Here's how the part is built. I have some questions about the finished solid (model axes, mm). Face numbers are marked on the shaded views. A direction names the side the tool comes from. Coordinates: 2 decimals unless noted, no trailing zeros. Loops run counter-clockwise (first coordinate to the right, second up) from the corner with the lowest first, then second, coordinate; pieces in that order, holes last. Notation, with made-up numbers: (-36.75, -16) -> (7.25, -16) arc R23 cw to (7.25, -4) -> close; hole circle Ø6 at (21.5, 50.5). An arc over 180 degrees is marked (long way). Use CSV: the item, a comma, the result in double quotes. Start each with the question number.
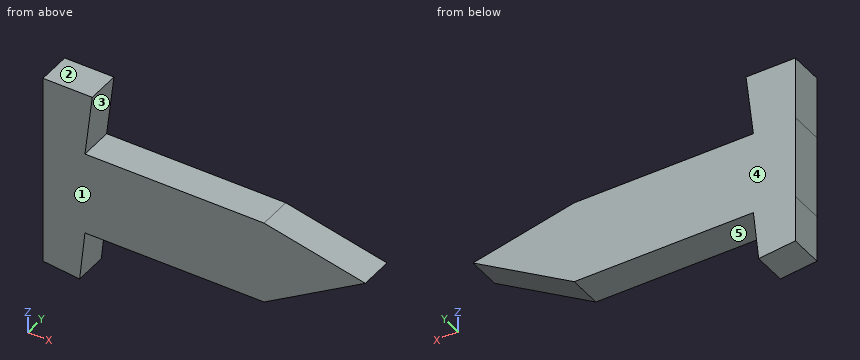
from build123d import *

# Parameters (mm, degrees)
F0_W     = 31.524651
F0_H     = 62.468918
F0_W_2   = 134.60525
F1_DEPTH = 25.4


with BuildPart() as f1:
    # F0 (on Front) → F1 (new body)
    with BuildSketch(Plane.XZ):
        with Locations((-136.606816, -14.502092)):
            Rectangle(F0_W, F0_H)
        Polygon((-120.844491, -45.736551), (-152.369142, -45.736551), (-152.369142, -80.935445), (-124.847621, -83.827771), align=None)
        with Locations((-53.541866, -14.502092)):
            Rectangle(F0_W_2, F0_H)
        Polygon((-152.369142, 63.859507), (-152.369142, 16.732367), (-120.844491, 16.732367), (-115.340188, 63.859507), align=None)
        Polygon((13.760759, 16.732367), (13.760759, -45.736551), (89.820236, 0), align=None)
    extrude(amount=F1_DEPTH)


solid = f1.part
1) I want a section at A-A, the plane y = -4.75. Please give me the cut outline in (x, z), plus the area to 3 significant figures.
2) Thinking about a two-plate mould opening in Z: for the marked faces 1, 2 and 3, which applies, pulls with the +Z half, pulls with the -Z half, needs draft (parallel to the pull), parting line crosses it, or undercut?
3) Which directions (+Z, -Z, +X, -X, +Y, -Y) give clear straight access to the entire face, cutting with the end or side of a thin tool? Please do the marked faces 4 and 5.
4) I want a section at B-B, the plane x = -40.5. Please give me the cut outline in (y, z), plus the area to 3 significant figures.
5) I want a section at C-C, the plane z = 12. Please give me the cut outline in (x, y), plus the area to 3 significant figures.
6) For P1, Ø4, axis at x = -51.5, y = -18, coming from the -Z side; P2, Ø1, axis at y = -14, z = -21, coming from the +X side; P3, Ø12, axis at y = -20, z = -9.5, coming from the +X side, each with a flat end and sliding along its axis, tell me the tip position at first contact or that it passes through.
7) Please list where these lines run through material, in increasing order: L1, parallel to Z at x = -64, y = -22.5; L2, parallel to X at y = -4.5, z = 44.5; L3, parallel to X at y = -12.75, z = 18. Write a range as [from, to].
Return value:
1,outline,"(-152.37, -80.94) -> (-124.85, -83.83) -> (-120.84, -45.74) -> (13.76, -45.74) -> (89.82, 0) -> (13.76, 16.73) -> (-120.84, 16.73) -> (-115.34, 63.86) -> (-152.37, 63.86) -> close"
1,area,"15,500 mm²"
2,face 1,"needs draft"
2,face 2,"pulls with the +Z half"
2,face 3,"undercut"
3,face 4,"+Z, -Z, +X, -X, +Y"
3,face 5,"-Z, +X, +Y, -Y"
4,outline,"(-25.4, -45.74) -> (0, -45.74) -> (0, 16.73) -> (-25.4, 16.73) -> close"
4,area,"1,590 mm²"
5,outline,"(-152.37, -25.4) -> (35.27, -25.4) -> (35.27, 0) -> (-152.37, 0) -> close"
5,area,"4,770 mm²"
6,P1,"stops at z = -45.74"
6,P2,"stops at x = 55.73"
6,P3,"stops at x = 84"
7,L1,"z = [-45.74, 16.73]"
7,L2,"x = [-152.37, -117.6]"
7,L3,"x = [-152.37, -120.7]"
